Answer from the drawing. Dimensions are ordinates in mm from the lowest x, y and z of the part. A direction names the side the tool comes from. Give positions to 0.01 mm unless a question says otherwise; leave off trailing zeros. Write each loop counter-clockwise with the first axis right and the second up, starting at its lowest first coordinate (ties: lowest second). Pieces come first, ordered by that corner, then holes. Notation, with made-up numbers: (45, 45.25) -> (69, 45.25) arc R14 ccw to (69, 59.25) -> close; hole circle Ø8 at (80, 44). An arc over 180 degrees is marked (long way). Put each result on its own line as item: value. Start each with the question number.
1) A cutting plane is placed at D-D (z = 0.8). Write down the section's boundary in (x, y) (1 decimal).
2) A cutting plane is placed at C-C (y = 7.5). Write down the section's boundary in (x, z).
3) For a pull along Y with two mould halves and no side action, classify the marked faces 1, 2 and 3 as released by +Y, released by -Y, zero draft, split by the parting line, or undercut.
4) A cutting plane is placed at B-B (z = 2.55). Write down the section's boundary in (x, y).
5) Find the intervals of material crossed by line 1 along Y through (x, z) = (1.7, 4.3); line 2 along Z through (x, y) = (2, 5.75); line 3 along X through (y, z) = (7.75, 2.75), in increasing order. Write a range as from..to.
6) A cutting plane is placed at A-A (x = 2.4). Write down the section's boundary in (y, z).
7) Flat-ended cylindrical pins translate along their axes: pin 1 Ø1 at (x, y) = (2, 4) entering from +Z; pin 2 Ø1 at (x, y) = (2, 10) entering from -Z; pin 3 Ø2 at (y, z) = (8, 0.5) entering from -X. Find the tip coordinate at first contact, or state that the pin passes through.
8) For the marked faces 4 and 5, determine the directions among +Z, -Z, +X, -X, +Y, -Y from which every point of the face is accessible in a straight line to the end or side of a thin tool.
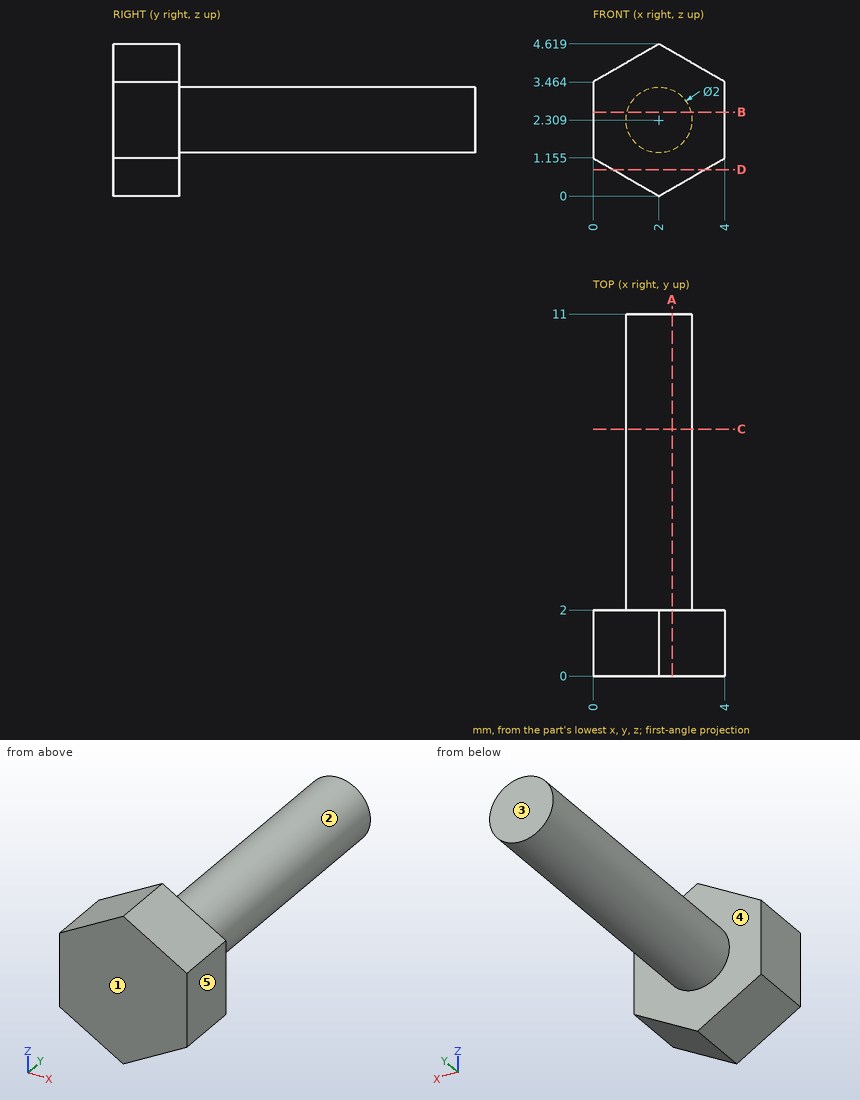
Reply:
1. outline: (0.6, 0) -> (3.4, 0) -> (3.4, 2) -> (0.6, 2) -> close
2. outline: circle Ø2 at (2, 2.31)
3. face 1: released by -Y
3. face 2: zero draft
3. face 3: released by +Y
4. outline: (0, 0) -> (4, 0) -> (4, 2) -> (2.97, 2) -> (2.97, 11) -> (1.03, 11) -> (1.03, 2) -> (0, 2) -> close
5. line 1: y = 0..2
5. line 2: z = 1.31..3.31
5. line 3: x = 1.1..2.9
6. outline: (0, 0.23) -> (2, 0.23) -> (2, 1.39) -> (11, 1.39) -> (11, 3.23) -> (2, 3.23) -> (2, 4.39) -> (0, 4.39) -> close
7. pin 1: stops at z = 3.31
7. pin 2: stops at z = 1.31
7. pin 3: stops at x = 1.41
8. face 4: +Y
8. face 5: +Z, -Z, +X, +Y, -Y
